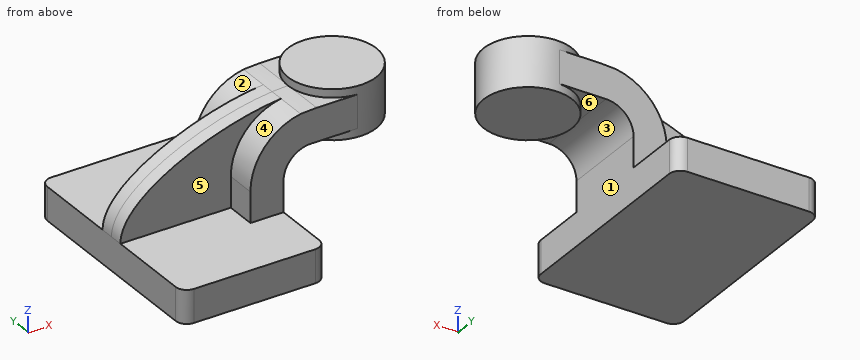
```python
from build123d import *

# Parameters (mm, degrees)
F1_DEPTH = 63.5
F0_W     = 25.332664
F0_H     = 19.05
F2_DEPTH = 25.4
F3_DEPTH = 7.9375
F5_R     = 6.35


with BuildPart() as f1:
    # F0 (on Front) → F1 (new body, symmetric)
    with BuildSketch(Plane.XZ):
        Polygon((-41.275, 9.525), (-41.275, -9.525), (41.275, -9.525), (41.275, 9.525), (22.225, 9.525), align=None)
    extrude(amount=F1_DEPTH, both=True)

    # F0 (on Front) → F2 (join, symmetric)
    with BuildSketch(Plane.XZ):
        with BuildLine():
            Line((22.225, 9.525), (41.275, 9.525))
            Line((41.275, 9.525), (41.275, 27.0002))
            ThreePointArc((41.275, 27.0002), (45.92468, 38.22552), (57.15, 42.8752))
            Line((57.15, 42.8752), (60.325, 42.8752))
            Line((60.325, 42.8752), (60.325, 61.9252))
            add(Edge.make_bspline(
                [(51.116651, 61.400117), (54.290802, 61.705885), (57.372222, 61.884054), (60.325, 61.9252)],
                knots=[105.745107, 105.745107, 105.745107, 105.745107, 114.316845, 114.316845, 114.316845, 114.316845], degree=3))
            ThreePointArc((51.116651, 61.400117), (30.406119, 49.461733), (22.225, 27.0002))
            Line((22.225, 27.0002), (22.225, 9.525))
        make_face()
        with Locations((72.991332, 52.4002)):
            Rectangle(F0_W, F0_H)
    extrude(amount=F2_DEPTH, both=True)

    # F0 (on Front) → F3 (join, symmetric)
    with BuildSketch(Plane.XZ):
        with BuildLine():
            add(Edge.make_bspline(
                [(-41.275, 9.525), (-41.311846, 34.437038), (11.958779, 57.628027), (51.116651, 61.400117)],
                knots=[0, 0, 0, 0, 105.745107, 105.745107, 105.745107, 105.745107], degree=3))
            Line((-41.275, 9.525), (22.225, 9.525))
            Line((22.225, 9.525), (22.225, 27.0002))
            ThreePointArc((22.225, 27.0002), (30.406119, 49.461733), (51.116651, 61.400117))
        make_face()
    extrude(amount=F3_DEPTH, both=True)

    # F0 (on Front) → F4 (revolve)
    with BuildSketch(Plane.XZ):
        Polygon((85.657664, 66.675), (85.657664, 61.9252), (85.657664, 42.8752), (85.657664, 38.1), (111.125, 38.1), (111.125, 66.675), align=None)
    revolve(axis=Axis((85.657664, 0, 52.3875), (0, 0, 1)))

    # F5
    f5_edges = [f1.edges().sort_by_distance(p)[0] for p in [
        (-41.275, -63.5, 0),
        (41.275, -63.5, 0),
        (41.275, 63.5, 0),
        (-41.275, 63.5, 0),
    ]]
    fillet(f5_edges, radius=F5_R)


solid = f1.part
```
Verification items for the finished model (mm, model axes). Face numbers are marked on the shaded views. A direction names the side the tool comes from. Coordinates: 2 decimals unless noted, no trailing zeros. Loops run counter-clockwise (first coordinate to the right, second up) from the corner with the lowest first, then second, coordinate; pieces in that order, holes last. Notation, with made-up numbers: (-36, 85.5) -> (-3, 85.5) arc R32 cw to (-3, 114.5) -> close; hole circle Ø9 at (-2, -34). An arc over 180 degrees is marked (long way). Answer in a Markdown table with one row per item. Add a question column.
1. Section check B-B, the plane x = 70.5. Enter the section's corners in (y, z) (3 decimals).
2. Material ranges on probe 1 along Y at (x, z) = (13, 41); probe 2 along Y at (x, z) = (50, 57); probe 3 along X at (y, z) = (55, -4.5) (3 decimals), recorded low to high. Write a range as [from, to].
3. Depth check by flat-ended pin: P1, Ø4, axis at x = 44, y = -10.5, coming from the +Z side; P2, Ø15.5, axis at x = -3, z = 25, coming from the -Y side; P3, Ø1, axis at x = 34, z = 32, coming from the -Y side. Enter the tip coordinate at first touch or a pass-through.
4. Access from +Z, -Z, +X, -X, +Y, -Y to the whole of each face (thin tool, end or side, straight path). Record for the marked faces 1 and 2.
5. Draft check along X on the marked faces 3, 4, 5 and 6. Enter one of: +X half, -X half, draft (parallel to the pull), parting line (faces both ways), or undercut.
6. Section check A-A, the plane y = -36.5. Enter the section's corners in (x, z) (3 decimals), then the cut area to 3 significant figures.
Derived:
| question | item | result |
|---|---|---|
| 1 | outline | (-25.4, 42.875) -> (-20.465, 42.875) -> (-20.465, 38.1) -> (20.465, 38.1) -> (20.465, 42.875) -> (25.4, 42.875) -> (25.4, 61.925) -> (20.465, 61.925) -> (20.465, 66.675) -> (-20.465, 66.675) -> (-20.465, 61.925) -> (-25.4, 61.925) -> close |
| 2 | probe 1 | y = [-7.94, 7.94] |
| 2 | probe 2 | y = [-25.4, 25.4] |
| 2 | probe 3 | x = [-41.275, 41.275] |
| 3 | P1 | stops at z = 60.1 |
| 3 | P2 | stops at y = -7.94 |
| 3 | P3 | stops at y = -25.4 |
| 4 | face 1 | -Z, +X, +Y, -Y |
| 4 | face 2 | +Z, -X, +Y |
| 5 | face 3 | undercut |
| 5 | face 4 | -X half |
| 5 | face 5 | draft |
| 5 | face 6 | undercut |
| 6 | outline | (-41.275, -9.525) -> (41.275, -9.525) -> (41.275, 9.525) -> (-41.275, 9.525) -> close |
| 6 | area | 1,570 mm² |
